```python
from build123d import *

# Parameters (mm, degrees)
ESQUISSE1_W             = 90
ESQUISSE1_H             = 2
BASE_EXTRUSION_DEPTH    = 264
ESQUISSE2_W             = 30
ESQUISSE2_H             = 22
ENL_V_MAT_EXTRU_1_DEPTH = 279.92651362
CONG_1_R                = 5
CHANFREIN1_SIZE         = 0.2
ESQUISSE3_R             = 1.7
ENL_V_MAT_EXTRU_2_DEPTH = 279.92651362


with BuildPart() as part:
    # Esquisse1 → Base-Extrusion (new body)
    with BuildSketch(Plane.XY):
        with Locations((45, 1)):
            Rectangle(ESQUISSE1_W, ESQUISSE1_H)
    extrude(amount=BASE_EXTRUSION_DEPTH)

    # Esquisse2 → Enlèv. mat.-Extru.1 (cut, through all)
    with BuildSketch(Plane(origin=(0, 2, 0), x_dir=(-1, 0, 0), z_dir=(0, 1, 0))):
        with Locations((-55, 41)):
            Rectangle(ESQUISSE2_W, ESQUISSE2_H)
    extrude(amount=-ENL_V_MAT_EXTRU_1_DEPTH, mode=Mode.SUBTRACT)

    # Congé1
    cong_1_edges = [part.edges().sort_by_distance(p)[0] for p in [
        (0, 1, 0),
        (0, 1, 264),
        (90, 1, 0),
        (90, 1, 264),
    ]]
    fillet(cong_1_edges, radius=CONG_1_R)

    # Chanfrein1
    chanfrein1_edges = [part.edges().sort_by_distance(p)[0] for p in [
        (0, 0, 132),
        (1.464466094, 0, 1.464466094),
        (1.464466094, 0, 262.535533906),
        (45, 0, 0),
        (45, 0, 264),
        (88.535533906, 0, 1.464466094),
        (88.535533906, 0, 262.535533906),
        (90, 0, 132),
        (70, 0, 41),
        (55, 0, 30),
        (40, 0, 41),
        (55, 0, 52),
        (0, 2, 132),
        (1.464466094, 2, 1.464466094),
        (1.464466094, 2, 262.535533906),
        (45, 2, 0),
        (45, 2, 264),
        (88.535533906, 2, 1.464466094),
        (88.535533906, 2, 262.535533906),
        (90, 2, 132),
        (70, 2, 41),
        (55, 2, 30),
        (40, 2, 41),
        (55, 2, 52),
    ]]
    chamfer(chanfrein1_edges, length=CHANFREIN1_SIZE)

    # Esquisse3 → Enlèv. mat.-Extru.2 (cut, through all)
    with BuildSketch(Plane(origin=(0, 2, 0), x_dir=(-1, 0, 0), z_dir=(0, 1, 0))):
        with Locations((-7.82, 251.51)):
            Circle(ESQUISSE3_R)
        with Locations((-7.82, 12.49)):
            Circle(ESQUISSE3_R)
        with Locations((-85, 252.5)):
            Circle(ESQUISSE3_R)
        with Locations((-85, 11.5)):
            Circle(ESQUISSE3_R)
    extrude(amount=-ENL_V_MAT_EXTRU_2_DEPTH, mode=Mode.SUBTRACT)


solid = part.part
```
Model file for the job. Use its own axes, mm. Coordinates: 2 decimals unless noted, no trailing zeros. Order: outer loops, then holes, each group sorted by start corner. A loop starts at its lowest first (then second) coordinate and runs counter-clockwise, first axis right, second up. Notation, with made-up numbers: (-29.75, 26) - (16.25, 26) arc R20 ccw to (16.25, 45) - close; hole circle Ø9 at (-6, 79). An arc over 180 degrees is marked (long way). Return JSON: item names as keys, results as strings. Group by question number.
1) Probe line 1 (Z direction, x = 7.82, y = 1.3); line 2 (Z direction, x = 85, y = 1); line 3 (Z direction, x = 54, y = 0.25). List the from-to ranges inside material, lowest first. Write a range as from..to.
2) Saw through at A-A, the plane x = 51. Write the cut outline in (y, z).
3) Saw through at B-B, the plane y = 1.1. Write the cut outline in (x, z).
4) Flat gauge pin, fed straight in: P1, Ø2.5, axis at x = 7.82, z = 251.51, coming from the +Y side. Where does the tip first touch, or does it go through?
Values found:
{
 "1": {"line 1": "z = 0..10.79, 14.19..249.81, 253.21..264", "line 2": "z = 0..9.8, 13.2..250.8, 254.2..264", "line 3": "z = 0..30, 52..264"},
 "2": {"outline": "(0, 0.2) - (0.2, 0) - (1.8, 0) - (2, 0.2) - (2, 29.8) - (1.8, 30) - (0.2, 30) - (0, 29.8) - close; (0, 52.2) - (0.2, 52) - (1.8, 52) - (2, 52.2) - (2, 263.8) - (1.8, 264) - (0.2, 264) - (0, 263.8) - close"},
 "3": {"outline": "(0, 5) arc R5 ccw to (5, 0) - (85, 0) arc R5 ccw to (90, 5) - (90, 259) arc R5 ccw to (85, 264) - (5, 264) arc R5 ccw to (0, 259) - close; hole circle Ø3.4 at (7.82, 12.49); hole circle Ø3.4 at (7.82, 251.51); hole (40, 30) - (70, 30) - (70, 52) - (40, 52) - close; hole circle Ø3.4 at (85, 11.5); hole circle Ø3.4 at (85, 252.5)"},
 "4": {"P1": "passes through"}
}
